The model under review builds one solid part; all positions refer to its coordinate system, in mm. A direction names the side the tool comes from. Coordinates: 2 decimals unless noted, no trailing zeros. Order: outer loops, then holes, each group sorted by start corner. A loop starts at its lowest first (then second) coordinate and runs counter-clockwise, first axis right, second up. Notation, with made-up numbers: M 65.25,30 L 98.25,30 A34 cw 98.25,60 Z; hole C 83,20 d5. An arc over 180 degrees is marked long. Write each question's results on one line, items separated by ' | '.
from build123d import *
from OCP.BRepFilletAPI import BRepFilletAPI_MakeChamfer

# Parameters (mm, degrees)
SKETCH1_W                       = 48.26
SKETCH1_H                       = 27.94
BOSS_EXTRUDE1_DEPTH             = 85.09
CUT_EXTRUDE1_DEPTH              = 82.55
F_43_0_089_DIAMETER_HOLE1_D     = 2.2606
F_43_0_089_DIAMETER_HOLE1_DEPTH = 19.05
F_43_0_089_DIAMETER_HOLE1_TIP   = 0.679152758
SKETCH4_W                       = 16.51
SKETCH4_H                       = 8.89
CUT_EXTRUDE2_DEPTH              = 88.13162629
CHAMFER1_SIZE                   = 3.81
FILLET1_R                       = 2.54
CHAMFER2_SIZE                   = 1.27
CHAMFER2_SIZE2                  = 0.889263574


with BuildPart() as part:
    # Sketch1 → Boss-Extrude1 (new body)
    with BuildSketch(Plane(origin=(0, 0, 0), x_dir=(1, 0, 0), z_dir=(0, 1, 0))):
        Rectangle(SKETCH1_W, SKETCH1_H)
    extrude(amount=BOSS_EXTRUDE1_DEPTH)

    # Sketch3 → Cut-Extrude1 (cut)
    with BuildSketch(Plane(origin=(0, 85.09, 0), x_dir=(1, 0, 0), z_dir=(0, 1, 0))):
        with BuildLine():
            Line((21.59, 0.508), (18.415, 0.508))
            Line((18.415, 0.508), (18.415, -4.572))
            Line((18.415, -4.572), (21.59, -4.572))
            Line((21.59, -4.572), (21.59, -6.35))
            Line((21.59, -6.35), (18.415, -6.35))
            Line((18.415, -6.35), (18.415, -11.43))
            Line((18.415, -11.43), (-18.415, -11.43))
            Line((-18.415, -11.43), (-18.415, -6.35))
            Line((-18.415, -6.35), (-21.59, -6.35))
            Line((-21.59, -6.35), (-21.59, -4.572))
            Line((-21.59, -4.572), (-18.415, -4.572))
            Line((-18.415, -4.572), (-18.415, 0.508))
            Line((-18.415, 0.508), (-21.59, 0.508))
            Line((-21.59, 0.508), (-21.59, 8.89))
            ThreePointArc((-21.59, 8.89), (-19.793948776, 9.633948776), (-19.05, 11.43))
            Line((-19.05, 11.43), (18.895098563, 11.43))
            ThreePointArc((18.895098563, 11.43), (19.694674714, 9.57999329), (21.59, 8.894727718))
            Line((21.59, 8.894727718), (21.59, 0.508))
        make_face()
    extrude(amount=-CUT_EXTRUDE1_DEPTH, mode=Mode.SUBTRACT)

    # #43 (0.089) Diameter Hole1
    with Locations(Plane(origin=(0, 85.09, 0), x_dir=(1, 0, 0), z_dir=(0, 1, 0))):
        with Locations((-21.59, 11.43), (21.59, 11.43), (21.59, -11.43), (-21.705255142, -11.683941121)):
            Hole(F_43_0_089_DIAMETER_HOLE1_D / 2, depth=F_43_0_089_DIAMETER_HOLE1_DEPTH)
            with Locations((0, 0, -(F_43_0_089_DIAMETER_HOLE1_DEPTH + F_43_0_089_DIAMETER_HOLE1_TIP / 2))):  # 118° drill point
                Cone(0, F_43_0_089_DIAMETER_HOLE1_D / 2, F_43_0_089_DIAMETER_HOLE1_TIP, mode=Mode.SUBTRACT)

    # Sketch4 → Cut-Extrude2 (cut, through all)
    with BuildSketch(Plane(origin=(0, 2.54, 0), x_dir=(1, 0, 0), z_dir=(0, 1, 0))):
        with Locations((0, -0.127)):
            Rectangle(SKETCH4_W, SKETCH4_H)
    extrude(amount=-CUT_EXTRUDE2_DEPTH, mode=Mode.SUBTRACT)

    # Chamfer1
    # the kernel refuses this chamfer: 3.81 mm, written as the material it takes off along each edge
    with BuildSketch(Plane(origin=(18.415, 94.888112184, -0.508), x_dir=(0.9996219169112968, 0, -0.027495876610586445), z_dir=(0, -1, 0))) as chamfer1_piece_1_section:
        Polygon((CHAMFER1_SIZE * 0.999621916911, CHAMFER1_SIZE * 0.0274958766106), (-CHAMFER1_SIZE * 0.0274958766106, CHAMFER1_SIZE * 0.999621916911), (0, 0), align=None)
    chamfer1_piece_1 = extrude(amount=92.348112184, mode=Mode.PRIVATE)
    chamfer1_piece_1 = split(chamfer1_piece_1, bisect_by=Plane(origin=(21.59, 43.815, 0.792238095), z_dir=(-1, 0, 0)), keep=Keep.TOP, mode=Mode.PRIVATE)
    add(chamfer1_piece_1, mode=Mode.SUBTRACT)
    with BuildSketch(Plane(origin=(-18.415, 94.888112184, -0.508), x_dir=(-0.9996219169112968, 0, -0.027495876610586247), z_dir=(0, -1, 0))) as chamfer1_piece_2_section:
        Polygon((CHAMFER1_SIZE * 0.999621916911, -CHAMFER1_SIZE * 0.0274958766106), (-CHAMFER1_SIZE * 0.0274958766106, -CHAMFER1_SIZE * 0.999621916911), (0, 0), align=None)
    chamfer1_piece_2 = extrude(amount=92.348112184, mode=Mode.PRIVATE)
    chamfer1_piece_2 = split(chamfer1_piece_2, bisect_by=Plane(origin=(-21.59, 43.815, 0.792238095), z_dir=(1, 0, 0)), keep=Keep.TOP, mode=Mode.PRIVATE)
    add(chamfer1_piece_2, mode=Mode.SUBTRACT)

    # Fillet1
    fillet1_edges = [part.edges().sort_by_distance(p)[0] for p in [
        (24.13, 42.545, 13.97),
        (-24.13, 42.545, 13.97),
        (-24.13, 42.545, -13.97),
        (24.13, 42.545, -13.97),
    ]]
    fillet(fillet1_edges, radius=FILLET1_R)

    # Chamfer2: one chamfer whose edges measure the first distance from different faces: ONE call of the kernel's chamfer builder (chamfer() names one face for all edges)
    chamfer2_edges_1 = [part.edges().sort_by_distance(p)[0] for p in [
        (0, 0, 13.97),
        (24.13, 0, 0),
        (-24.13, 0, 0),
        (0, 0, -13.97),
        (-23.386051224, 0, -13.226051224),
        (23.386051224, 0, -13.226051224),
        (23.386051224, 0, 13.226051224),
        (-23.386051224, 0, 13.226051224),
    ]]
    chamfer2_side_1 = [part.faces().sort_by_distance(p)[0] for p in [
        (0, 0, 13.412355741),
    ]]
    chamfer2_edges_2 = [part.edges().sort_by_distance(p)[0] for p in [
        (8.255, 0, 0.127),
    ]]
    chamfer2_side_2 = [part.faces().sort_by_distance(p)[0] for p in [
        (8.255, 1.27, 0.127),
    ]]
    chamfer2_edges_3 = [part.edges().sort_by_distance(p)[0] for p in [
        (0, 0, 4.572),
    ]]
    chamfer2_side_3 = [part.faces().sort_by_distance(p)[0] for p in [
        (0, 1.27, 4.572),
    ]]
    chamfer2_edges_4 = [part.edges().sort_by_distance(p)[0] for p in [
        (-8.255, 0, 0.127),
    ]]
    chamfer2_side_4 = [part.faces().sort_by_distance(p)[0] for p in [
        (-8.255, 1.27, 0.127),
    ]]
    chamfer2_edges_5 = [part.edges().sort_by_distance(p)[0] for p in [
        (0, 0, -4.318),
    ]]
    chamfer2_side_5 = [part.faces().sort_by_distance(p)[0] for p in [
        (0, 1.27, -4.318),
    ]]
    chamfer2 = BRepFilletAPI_MakeChamfer(part.part.solid().wrapped)
    for e in chamfer2_edges_1:
        chamfer2.Add(CHAMFER2_SIZE, CHAMFER2_SIZE2, e.wrapped, chamfer2_side_1[0].wrapped)  # the first distance lies on this face
    for e in chamfer2_edges_2:
        chamfer2.Add(CHAMFER2_SIZE, CHAMFER2_SIZE2, e.wrapped, chamfer2_side_2[0].wrapped)  # the first distance lies on this face
    for e in chamfer2_edges_3:
        chamfer2.Add(CHAMFER2_SIZE, CHAMFER2_SIZE2, e.wrapped, chamfer2_side_3[0].wrapped)  # the first distance lies on this face
    for e in chamfer2_edges_4:
        chamfer2.Add(CHAMFER2_SIZE, CHAMFER2_SIZE2, e.wrapped, chamfer2_side_4[0].wrapped)  # the first distance lies on this face
    for e in chamfer2_edges_5:
        chamfer2.Add(CHAMFER2_SIZE, CHAMFER2_SIZE2, e.wrapped, chamfer2_side_5[0].wrapped)  # the first distance lies on this face
    add(Compound.cast(chamfer2.Shape()), mode=Mode.REPLACE)


solid = part.part
1) The part is to be moulded in two halves that separate along Z. For faces 1 (the conical face through (-22.857, 0.352, 12.67)), 2 (the conical face through (21.445, 65.479, -11.563)), 3 (the flat face through (20.025, 44.393, 1.692)), 4 (the flat face through (0, 42, -13.97)), say which applies: pulls with the +Z half, pulls with the -Z half, needs draft (parallel to the pull), parting line crosses it, or undercut.
Solutions:
face 1: pulls with the +Z half | face 2: undercut | face 3: undercut | face 4: pulls with the -Z half
2) Take a section at C-C on z = 1.5. State the section outline as (x, y) points (3 decimals), plus the area to 3 significant figures.
Solutions:
outline: M -24.13,0.889 L -22.86,0 L -9.144,0 L -8.255,1.27 L -8.255,2.54 L -20.217,2.54 L -20.217,85.09 L -24.13,85.09 Z; M 8.255,1.27 L 9.144,0 L 22.86,0 L 24.13,0.889 L 24.13,85.09 L 20.217,85.09 L 20.217,2.54 L 8.255,2.54 Z | area: 724 mm2
3) Take a section at D-D on x = -13.5. State the section outline as (y, z) points.
Solutions:
outline: M 0,-12.7 L 0.89,-13.97 L 85.09,-13.97 L 85.09,-11.43 L 2.54,-11.43 L 2.54,11.43 L 85.09,11.43 L 85.09,13.97 L 0.89,13.97 L 0,12.7 Z
4) Take a section at B-B on x = 6. State the section outline as (y, z) points.
Solutions:
outline: M 0,-12.7 L 0.89,-13.97 L 85.09,-13.97 L 85.09,-11.43 L 2.54,-11.43 L 2.54,-4.32 L 1.27,-4.32 L 0,-5.21 Z; M 0,5.46 L 1.27,4.57 L 2.54,4.57 L 2.54,11.43 L 85.09,11.43 L 85.09,13.97 L 0.89,13.97 L 0,12.7 Z
5) For faces 5 (the cylindrical face through (-23.406, 43.579, -13.206)), 6 (the flat face through (20, 44, 6.35)), list the 3-axis set-ups (+Z, -Z, +X, -X, +Y, -Y) from which the entire face can be reached by the end or side of a thin tool; tool diameter is ignored.
Solutions:
face 5: -Z, -X, +Y, -Y | face 6: +Y
6) To check wall thickness, follow line 1 along X through (y, z) = (54, 9.5) (3 decimals); line 2 along Z through (x, y) = (17, 73); line 3 along X through (y, z) = (30.5, 6.25). State the ranges of each line that lie inside material, in increasing order.
Solutions:
line 1: -24.13 to -18.415, 18.415 to 24.13 | line 2: -13.97 to -11.43, 11.43 to 13.97 | line 3: -24.13 to -21.59, 21.59 to 24.13
7) Take a section at A-A on y = 11.5. State the section outline as (x, z) points (3 decimals), plus the area to 3 significant figures.
Solutions:
outline: M -24.13,-11.43 A2.54 ccw -21.59,-13.97 L 21.59,-13.97 A2.54 ccw 24.13,-11.43 L 24.13,11.43 A2.54 ccw 21.59,13.97 L -21.59,13.97 A2.54 ccw -24.13,11.43 Z; hole M -21.59,-8.89 A2.54 cw -19.05,-11.43 L 18.895,-11.43 A2.54 cw 21.59,-8.895 L 21.59,0.127 L 18.415,3.302 L 18.415,4.572 L 21.59,4.572 L 21.59,6.35 L 18.415,6.35 L 18.415,11.43 L -18.415,11.43 L -18.415,6.35 L -21.59,6.35 L -21.59,4.572 L -18.415,4.572 L -18.415,3.302 L -21.59,0.127 Z | area: 417 mm2
8) For pin 1 (5 mm diameter, centred on x = 13, z = 2, fed in from +Y), flat-tipped, find the tip position at first contact; note if it passes through.
Solutions:
pin 1: y = 2.54
